Autodesk Inventor part; units mm, degrees
ref_plane "Plano de trabajo1" through (-63.7586, -34.3586, 1.8) normal (0, 0, -1) x (0, 1, 0)
ref_plane "Plano de trabajo2" through (-63.7586, -34.3586, 13.8) normal (0, 0, -1) x (0, 1, 0)
ref_plane "Plano de trabajo4" through (-58.0586, -29.3586, 1.8) normal (0, 0, 1) x (1, 0, 0)
sketch "Boceto2" plane through (0, 0, 0) normal (0, 0, 1) x (1, 0, 0)
  circle A0 centre (60.5, -11.7293) radius 1.25
  circle A1 centre (60.5, -32) radius 1.25
  line L0 (-63.5, 34.5) -> (63.5, 34.5)
  line L1 (-63.5, -34.5) -> (-63.5, 34.5)
  line L2 (63.5, -34.5) -> (-63.5, -34.5)
  line L3 (63.5, 34.5) -> (63.5, -34.5)
  line L4 (-37.2586, -7.2586) -> (-37.2586, -29.3586)
  line L5 (-58.4586, -34.5586) -> (-60.3586, -34.5586)
  line L6 (-70.2586, -17.8586) -> (-70.2586, -21.2586)
  line L7 (-60.3586, -2.2586) -> (-58.4586, -2.2586)
  line L8 (-58.4586, -2.2586) -> (-58.4586, -34.3586)
  line L9 (-60.3586, -34.3586) -> (-60.3586, -29.3586)
  line L10 (-60.5586, -2.2586) -> (-60.5586, -6.8586)
  line L11 (-60.5586, -2.2586) -> (-63.5, -2.2586)
  line L12 (-63.5, -2.2586) -> (-63.5, -34.5)
  line L13 (-63.5, -34.5) -> (-60.5586, -34.5)
  line L14 (-60.5586, -34.5) -> (-60.5586, -2.2586)
  circle A2 centre (-49.0086, -4.2586) radius 1
  circle A3 centre (-34.4586, -18.4086) radius 1
  point P0 (0, 0)
ref_plane "Plano de trabajo1" through (-63.7586, -34.3586, 1.8) normal (0, 0, -1) x (0, 1, 0)
extrude "Extrusión1" add sketch "Boceto2" along normal up to surface (1.8 mm away) contours L11 L10 L14 L2 L1
sketch "Boceto3" plane through (-63.5, -34.5, 1.8) normal (0, 0, 1) x (1, 0, 0)
  line L0 (2.9414, 4.9414) -> (-0.2586, 4.9414)
  line L1 (-0.0586, 27.4414) -> (2.7414, 27.4414)
  line L2 (-0.0586, 27.4414) -> (2.9414, 27.4414)
  line L3 (2.9414, 27.4414) -> (2.9414, 32.2414)
  line L4 (2.9414, 32.2414) -> (-0.0586, 32.2414)
  line L5 (-0.0586, 32.2414) -> (-0.0586, 27.4414)
  line L6 (-0.2586, 4.9414) -> (2.9414, 4.9414)
  line L7 (2.9414, 4.9414) -> (2.9414, 0)
  line L8 (2.9414, 0) -> (-0.2586, 0)
  line L9 (-0.2586, 0) -> (-0.2586, 4.9414)
  point P0 (63.5, 34.5)
ref_plane "Plano de trabajo2" through (-63.7586, -34.3586, 13.8) normal (0, 0, -1) x (0, 1, 0)
extrude "Extrusión2" add sketch "Boceto3" along normal up to surface (12 mm away)
sketch "Boceto4" plane through (-63.5586, -7.0586, 1.8) normal (-1, 0, 0) x (0, 0, 1)
  arc A0 (5.3, 3.7247) -> (6.7, 3.7247) centre (6, 2.75) ccw
  arc A1 (6.5, -26.3409) -> (5.3, -26.2247) centre (6, -25.25) ccw
  arc A2 (6.5, -26.3409) -> (5.3, -26.2247) centre (6, -25.25) ccw
  arc A3 (6.5, -26.3409) -> (5.3, -26.2247) centre (6, -25.25) ccw
  point P0 (-1.8, 7.0586)
hole "Agujero1" at (-63.5586, -4.3086, 7.8) direction (1, 0, 0) diameter 2 end up to surface
sketch "Boceto5" plane through (-63.7586, -34.5, 1.8) normal (-1, 0, 0) x (0, 0, 1)
  arc A0 (6.5, 1.1006) -> (5.3, 1.2167) centre (6, 2.1914) ccw
  point P0 (-1.8, 34.5)
hole "Agujero2" at (-63.7586, -32.3086, 7.8) direction (1, 0, 0) diameter 2 end up to surface
move faces "Desplazar1" translate (-0.0586, 0, 0) faces at (-63.5, -14.6057, 0.6)
move faces "Desplazar2" translate (0.2, 0, 0) faces at (-63.7586, -32.1224, 3.4667)
ref_plane "Plano de trabajo3" through (0, 0, 0) normal (0, 0, 1) x (1, 0, 0)
sketch "Boceto6" plane through (0, 0, 0) normal (0, 0, 1) x (1, 0, 0)
  line L0 (-37.4586, -7.2586) -> (-37.4586, -29.3586)
  line L1 (-37.4586, -29.3586) -> (-37.4586, -38.3484)
  circle A0 centre (60.5, -11.7293) radius 1.25
  circle A1 centre (60.5, -32) radius 1.25
  line L2 (-63.5, 34.5) -> (63.5, 34.5)
  line L3 (-63.5, -34.5) -> (-63.5, 34.5)
  line L4 (63.5, -34.5) -> (-63.5, -34.5)
  line L5 (63.5, 34.5) -> (63.5, -34.5)
  line L6 (-58.0586, -7.2586) -> (-37.4586, -7.2586)
  line L7 (-58.0586, -29.5586) -> (-37.4586, -29.5586)
  line L8 (-37.4586, -29.5586) -> (-60.5586, -29.5586)
  line L9 (-60.5586, -34.5) -> (-60.5586, -2.2586)
  line L10 (-60.5586, -29.5586) -> (-37.4586, -29.5586)
  line L11 (-37.4586, -29.5586) -> (-37.4586, -7.2586)
  line L12 (-37.4586, -7.2586) -> (-60.5586, -7.2586)
  line L13 (-60.5586, -7.2586) -> (-60.5586, -29.5586)
  circle A2 centre (-49.0086, -4.2586) radius 1
  circle A3 centre (-34.4586, -18.4086) radius 1
  point P0 (0, 0)
ref_plane "Plano de trabajo4" through (-58.0586, -29.3586, 1.8) normal (0, 0, 1) x (1, 0, 0)
extrude "Extrusión3" add sketch "Boceto6" along normal up to surface (1.8 mm away) contours L0 L1 L7 L8 L9 L12 L6
sketch "Boceto7" plane through (-37.4586, -29.5586, 0) normal (1, 0, 0) x (0, 0, -1)
  line L0 (-1.8, 0) -> (-1.8, 22.3)
  line L1 (-1.8, 22.3) -> (-1.8, 0)
  line L2 (-1.8, 11.15) -> (0, 11.15)
  line L3 (0, 0) -> (0, 22.3)
  line L4 (0, 8.15) -> (-1.8, 8.15)
  line L5 (-1.8, 8.15) -> (-1.8, 14.15)
  line L6 (-1.8, 14.15) -> (0, 14.15)
  line L7 (0, 14.15) -> (0, 8.15)
  line L8 (0, 8.15) -> (-1.8, 14.15) construction
  line L9 (-1.8, 8.15) -> (0, 14.15) construction
  point P0 (0, 29.5586)
  point P1 (-0.9, 11.15)
  dimension "d26" = 6
extrude "Extrusión4" add sketch "Boceto7" along normal blind 6
sketch "Boceto8" plane through (-63.5586, -7.0586, 1.8) normal (0, 0, 1) x (1, 0, 0)
  line L0 (26.1, -14.35) -> (26.1, -8.35)
  line L1 (26.1, -14.35) -> (29.1, -14.35)
  line L2 (26.1, -14.35) -> (32.1, -14.35)
  line L3 (26.1, -8.35) -> (32.1, -8.35)
  line L4 (29.1, -8.35) -> (29.1, -14.35)
  arc A0 (29.1, -14.35) -> (29.1, -8.35) centre (29.1, -11.35) ccw
  line L5 (32.1, -14.35) -> (32.1, -8.35)
  line L6 (29.1, -8.35) -> (32.0071, -8.35)
  line L7 (29.1, -14.35) -> (32.1, -14.35)
  point P0 (63.5586, 7.0586)
ref_plane "Plano de trabajo5" through (-63.5, -34.5, 0) normal (0, 0, 1) x (1, 0, 0)
extrude "Extrusión5" cut sketch "Boceto8" against normal up to surface (1.8 mm away) contours A0 L5 L2 | L3 L5 A0
hole "Agujero3" at (-34.4586, -18.4086, 1.8) direction (0, 0, -1) diameter 2 depth 1.8 tip angle 118
sketch "Boceto10" plane through (-60.5586, -7.2586, 0) normal (0, 1, 0) x (1, 0, 0)
  line L0 (23.1, 0) -> (0, 0)
  line L1 (11.55, 0) -> (11.55, -1.8)
  line L2 (0, -1.8) -> (23.1, -1.8)
  line L3 (14.55, -1.8) -> (8.55, -1.8)
  line L4 (8.55, -1.8) -> (8.55, 0)
  line L5 (8.55, 0) -> (14.55, 0)
  line L6 (14.55, 0) -> (14.55, -1.8)
  line L7 (14.55, -1.8) -> (8.55, 0) construction
  line L8 (8.55, -1.8) -> (14.55, 0) construction
  point P0 (60.5586, 0)
  point P1 (11.55, -0.9)
  dimension "d40" = 6
extrude "Extrusión6" add sketch "Boceto10" along normal blind 6
sketch "Boceto11" plane through (-63.5586, -7.0586, 1.8) normal (0, 0, 1) x (1, 0, 0)
  line L0 (17.55, -0.2) -> (17.55, 5.8)
  line L1 (17.55, 2.8) -> (11.55, 2.8)
  line L2 (11.55, -0.2) -> (11.55, 5.8)
  arc A0 (17.55, 2.8) -> (11.55, 2.8) centre (14.55, 2.8) ccw
  line L3 (17.55, 5.8) -> (11.55, 5.8)
  line L4 (11.55, 2.8) -> (11.55, 5.8)
  line L5 (11.55, 5.8) -> (17.55, 5.8)
  line L6 (17.55, 2.8) -> (17.55, 5.8)
  point P0 (63.5586, 7.0586)
ref_plane "Plano de trabajo6" through (-63.5, -34.5, 0) normal (0, 0, 1) x (1, 0, 0)
extrude "Extrusión7" cut sketch "Boceto11" against normal up to surface (1.8 mm away) contours A0 L3 L0 | L2 L3 A0
hole "Agujero4" at (-49.0086, -4.2586, 1.8) direction (0, 0, -1) diameter 2 depth 1.8 tip angle 118
fillet "Empalme1" radius 5 1 edges at (-60.5586, -29.5586, 0.9)
properties part number "soporteIzq"
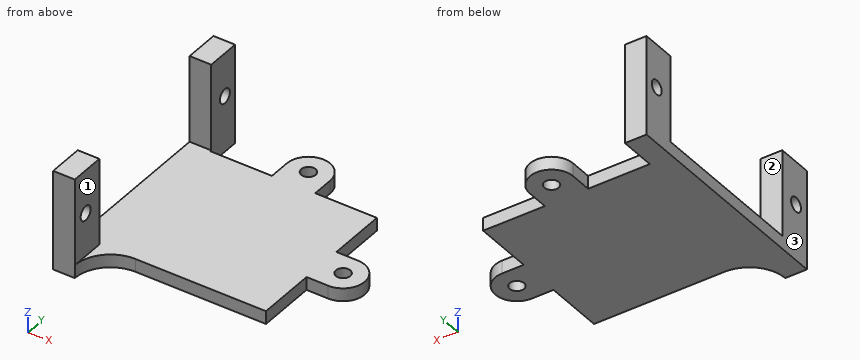
Work out the finished part from the listing and answer in its coordinate system (mm). Face numbers are marked on the shaded views. A direction names the side the tool comes from. Give positions to 0.01 mm unless a question says otherwise; leave off trailing zeros. Loops run counter-clockwise (first coordinate to the right, second up) from the corner with the lowest first, then second, coordinate; pieces in that order, holes last. Notation, with made-up numbers: M 82,-39 L 102,-39 A23 ccw 102,-5 Z; hole C 63,5.5 d5. An arc over 180 degrees is marked long. One line per item, written item: value. Start each with the question number.
1. Find section A-A (z = 7.8). Give the vertices of the cut face in (x, y), and give its area (3 significant figures).
2. Find section D-D (x = -40). Give the vertices of the cut face in (y, z), and give its area (3 significant figures).
3. Each of these flat-tipped pins is pushed along its axis until it touches: P1, Ø1.4, axis at x = -35.5, z = 0.5, coming from the +Y side; P2, Ø1.4, axis at x = -43.5, z = 0.5, coming from the +Y side; P3, Ø8, axis at x = -39, z = 8, coming from the -Y side; P4, Ø6, axis at x = -48, y = -9.5, coming from the -Z side. Where does it stop, or does it pass through?
4. Find section C-C (y = -13). Give the vertices of the cut face in (x, z), and give its area (3 significant figures).
5. Find section B-B (z = 2.75). Give the vertices of the cut face in (x, y), and give its area (3 significant figures).
6. Which of the six approach directions +Z, -Z, +X, -X, +Y, -Y give full straight-line access (tool end or side, diameter ignored) to the marked faces 1, 2 and 3?
7. Find the intervals of material crossed by probe 1 along Y at (x, z) = (-62.2, 7.8); probe 2 along Z at (x, y) = (-39.5, -24); probe 3 along X at (y, z) = (-10, 0.75), in increasing order.
Reported:
1. outline: M -63.56,-34.5 L -60.56,-34.5 L -60.56,-33.31 L -63.56,-33.31 Z; M -63.56,-31.31 L -60.56,-31.31 L -60.56,-29.56 L -63.56,-29.56 Z; M -63.56,-7.06 L -60.56,-7.06 L -60.56,-5.31 L -63.56,-5.31 Z; M -63.56,-3.31 L -60.56,-3.31 L -60.56,-2.26 L -63.56,-2.26 Z
1. area: 17.2 mm²
2. outline: M -29.56,0 L -7.26,0 L -7.26,1.8 L -29.56,1.8 Z
2. area: 40.1 mm²
3. P1: stops at y = -15.41
3. P2: stops at y = -7.26
3. P3: passes through
3. P4: stops at z = 0
4. outline: M -63.56,0 L -37.46,0 L -37.46,1.8 L -63.56,1.8 Z
4. area: 47.0 mm²
5. outline: M -63.56,-34.5 L -60.56,-34.5 L -60.56,-29.56 L -63.56,-29.56 Z; M -63.56,-7.06 L -60.56,-7.06 L -60.56,-2.26 L -63.56,-2.26 Z
5. area: 29.2 mm²
6. face 1: +Z, +X, +Y, -Y
6. face 2: +Z, +X, -X
6. face 3: +Z, -Z, -X, +Y, -Y
7. probe 1: y = -34.5 to -33.31, -31.31 to -29.56, -7.06 to -5.31, -3.31 to -2.26
7. probe 2: z = 0 to 1.8
7. probe 3: x = -63.56 to -37.46
